Source: three-view drawing plus pictorial views. Frame: mm from the lowest corner of the part. A direction names the side the tool comes from. Coordinates: 2 decimals unless noted, no trailing zeros. One line per question, with ' | ' between items.
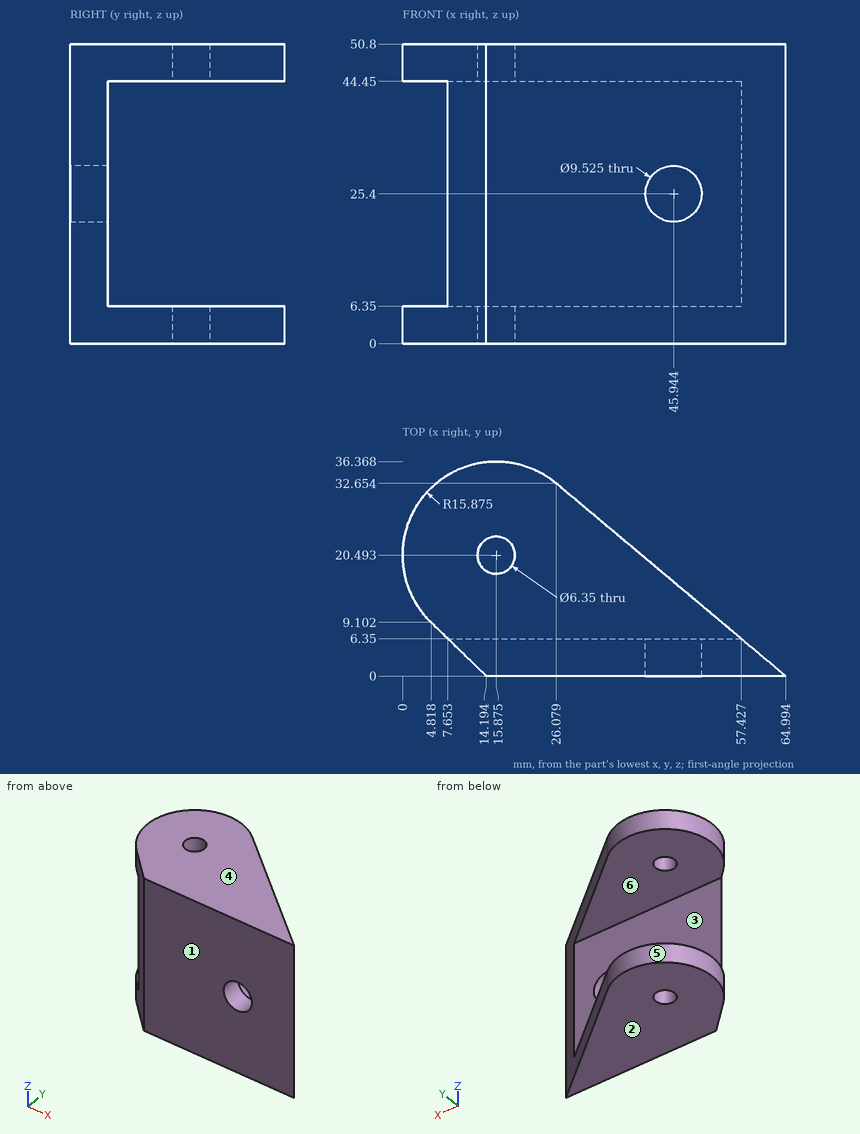
(1) Pull-direction query (Z, two-part tool) for the marked faces 1, 2, 3 and 4; classes: pulls with the +Z half, pulls with the -Z half, needs draft (parallel to the pull), parting line crosses it, or undercut.
Taken from the geometry:
face 1: needs draft | face 2: pulls with the -Z half | face 3: undercut | face 4: pulls with the +Z half
(2) Pin query (flat end, axial travel): P1, Ø10, axis at x = 15.88, y = 20.49, coming from the +Z side; P2, Ø2, axis at y = 17, z = 44, coming from the -X side; P3, Ø4, axis at y = 27.5, z = 8, coming from the -X side; P4, Ø6, axis at x = 56.5, z = 11.5, coming from the +Y side. Return the tip coordinate at first contact, or that it passes through.
Taken from the geometry:
P1: stops at z = 50.8 | P2: stops at x = 0.21 | P3: stops at x = 1.13 | P4: stops at y = 6.35
(3) Material intervals for L1, parallel to Z at x = 23, y = 13.5; L2, parallel to Y at x = 25, z = 39; L3, parallel to Y at x = 17.5, z = 46.5 (1 decimal), sorted ascending. Write a range as from..to.
Taken from the geometry:
L1: z = 0..6.35, 44.45..50.8 | L2: y = 0..6.35 | L3: y = 0..17.8, 23.2..36.3
(4) Set-up query: the marked faces 5 and 6. Return all of +Z, -Z, +X, -X, +Y, -Y with unobstructed straight access to the full face (end or side cutting, diameter ignored); none if empty.
Taken from the geometry:
face 5: +Z, -Z | face 6: +X, -X, +Y
